Design review of the part shown in the three views and the two pictorial views. Dimensions are in mm from the part's minimum x, y and z. A direction names the side the tool comes from. Coordinates: 2 decimals unless noted, no trailing zeros. Write each loop counter-clockwise with the first axis right and the second up, starting at its lowest first coordinate (ties: lowest second). Pieces come first, ordered by that corner, then holes. Notation, with made-up numbers: (-29, 76.5) -> (-2, 76.5) arc R17 ccw to (-2, 109.5) -> close; hole circle Ø3 at (53.5, -14). An arc over 180 degrees is marked (long way). Answer in a Markdown table with one row per item. Add a question column.
Item 1: Clearance check with flat-ended pins moving along their axes: P1, Ø1.8, axis at x = 14, z = 12, coming from the +Y side; P2, Ø5, axis at x = 14, z = 11, coming from the -Y side; P3, Ø1.8, axis at x = 17, z = 17, coming from the -Y side. State where each tip first meets the part, or that it passes through.
Item 2: Draft analysis for pull direction Z (two halves, no side actions). For the marked faces 1, 2 and 3, state which applies: released by +Z, released by -Z, zero draft, split by the parting line, or undercut.
Item 3: To check wall thickness, follow line 1 (Y direction, x = 9.8, z = 0.7); line 2 (X direction, y = 1.9, z = 23.5); line 3 (X direction, y = 1.9, z = 17). State the ranges of each line that lie inside material, in increasing order.
Item 4: For the marked faces 4 and 5, list the 3-axis set-ups (+Z, -Z, +X, -X, +Y, -Y) from which the entire face can be reached by the end or side of a thin tool; tool diameter is ignored.
Item 5: Take a section at C-C, the plane z = 11. Write out the cut boundary in (x, y).
Item 6: Take a section at A-A, the plane z = 23.5. Write out the cut boundary in (x, y).
Item 7: Take a section at B-B, the plane x = 9.8. Write out the cut boundary in (y, z).
Item 8: Take a section at D-D, the plane x = 14.8. Write out the cut boundary in (y, z), and give its area (3 significant figures).
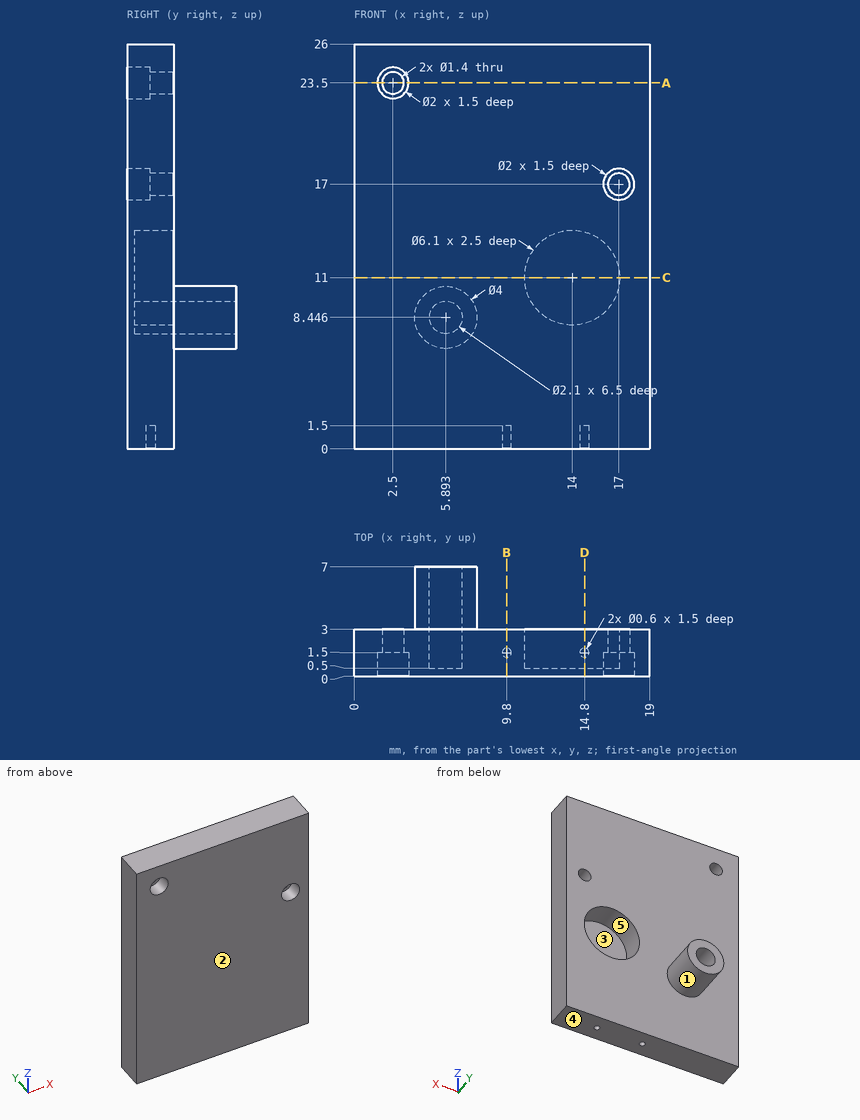
Answers:
| question | item | result |
|---|---|---|
| 1 | P1 | stops at y = 0.5 |
| 1 | P2 | stops at y = 0 |
| 1 | P3 | stops at y = 1.5 |
| 2 | face 1 | split by the parting line |
| 2 | face 2 | zero draft |
| 2 | face 3 | undercut |
| 3 | line 1 | y = 0 to 1.2, 1.8 to 3 |
| 3 | line 2 | x = 0 to 1.8, 3.2 to 19 |
| 3 | line 3 | x = 0 to 16.3, 17.7 to 19 |
| 4 | face 4 | -Z, +X, -X, +Y, -Y |
| 4 | face 5 | +Y |
| 5 | outline | (0, 0) -> (19, 0) -> (19, 3) -> (17.05, 3) -> (17.05, 0.5) -> (10.95, 0.5) -> (10.95, 3) -> (0, 3) -> close |
| 6 | outline | (0, 0) -> (1.5, 0) -> (1.5, 1.5) -> (1.8, 1.5) -> (1.8, 3) -> (0, 3) -> close; (3.2, 1.5) -> (3.5, 1.5) -> (3.5, 0) -> (19, 0) -> (19, 3) -> (3.2, 3) -> close |
| 7 | outline | (0, 0) -> (1.2, 0) -> (1.2, 1.5) -> (1.8, 1.5) -> (1.8, 0) -> (3, 0) -> (3, 26) -> (0, 26) -> close |
| 8 | outline | (0, 0) -> (1.2, 0) -> (1.2, 1.5) -> (1.8, 1.5) -> (1.8, 0) -> (3, 0) -> (3, 8.06) -> (0.5, 8.06) -> (0.5, 13.94) -> (3, 13.94) -> (3, 26) -> (0, 26) -> close |
| 8 | area | 62.4 mm^2 |
